Geometry: see drawing. Coordinates: mm, zero at the bounding-box minimum. Round coordinates to 2 decimals unless told otherwise and drop trailing zeros. Write each loop counter-clockwise with the first axis right and the second up, starting at its lowest first coordinate (ties: lowest second). Pieces come first, ordered by that corner, then holes. Notation, with made-up numbers: M 75.5,47.25 L 132.5,47.25 A21 cw 132.5,52.25 Z; hole C -28.75,-25 d2. An arc over 180 degrees is marked long. Use one line per item in the form item = value. Start each with the question number.
Item 1: Section query B-B (x = 95). Return loops of the section in (y, z), and give its area (3 significant figures).
Item 2: Ray query, probe 1 along Z at (x, y) = (225, 7.5); probe 2 along Z at (x, y) = (148.5, 4.75); probe 3 along X at (y, z) = (10, 190). Return the intervals inside material, ascending.
Item 3: Pin query (flat end, axial travel): pin 1 Ø1 at (x, y) = (99.5, 5) entering from -Z; pin 2 Ø2 at (y, z) = (4, 185) entering from -X; pin 3 Ø6 at (x, y) = (7, 5.5) entering from -Z; pin 4 Ø3.5 at (x, y) = (8, 5.5) entering from +Z. Return the tip coordinate at first contact, or that it passes through.
Item 4: Section query A-A (z = 54). Return loops of the section in (x, y).
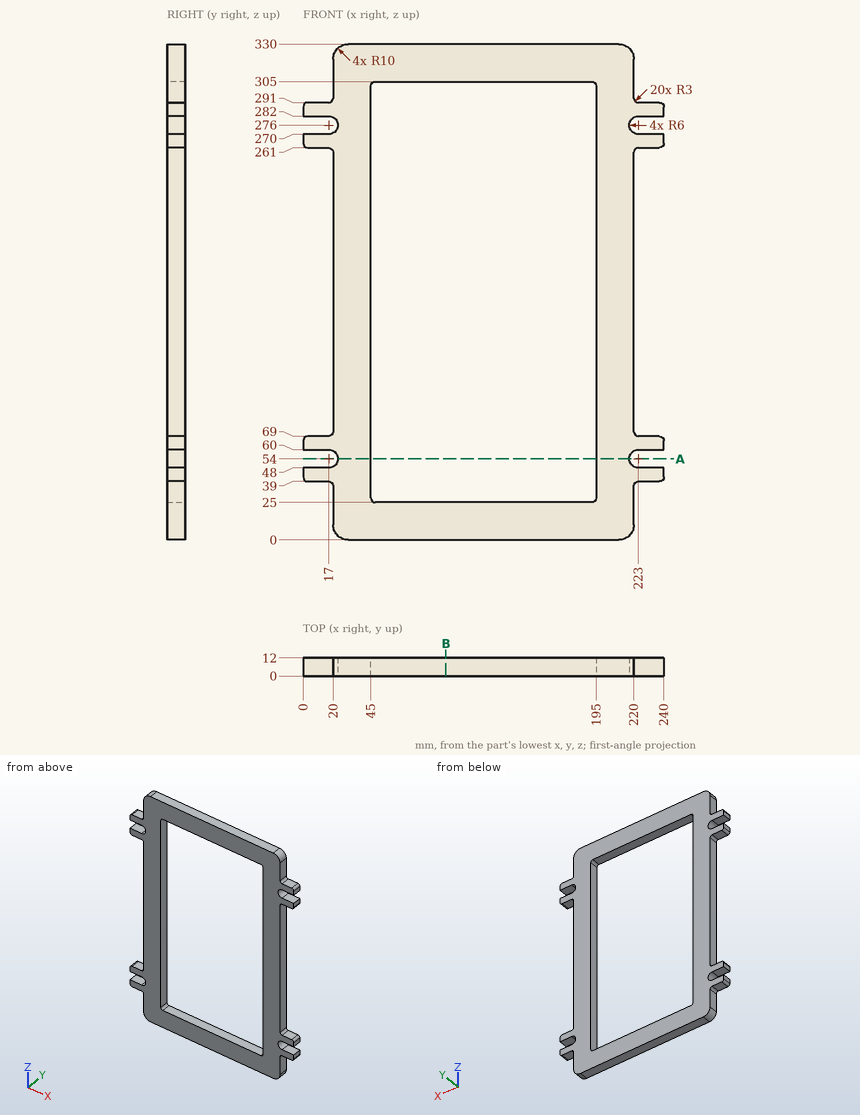
Working result:
q1.outline = M 0,0 L 12,0 L 12,25 L 0,25 Z; M 0,305 L 12,305 L 12,330 L 0,330 Z
q1.area = 600 mm²
q2.probe_1 = 39 to 48, 60 to 69, 261 to 270, 282 to 291
q2.probe_2 = 0 to 25, 305 to 330
q2.probe_3 = 20 to 45, 195 to 220
q3.pin_1 = 0
q3.pin_2 = 20
q3.pin_3 = 39
q3.pin_4 = 291
q4.outline = M 23,0 L 45,0 L 45,12 L 23,12 Z; M 195,0 L 217,0 L 217,12 L 195,12 Z
